from build123d import *

# Parameters (mm, degrees)
SKETCH1_R               = 2.2098
BOSS_EXTRUDE1_DEPTH     = 12.573
CUT_EXTRUDE1_DEPTH      = 3.429
CUT_EXTRUDE1_DEPTH_BACK = 59.054456093
CUT_EXTRUDE5_DEPTH      = 59.054456093
CUT_EXTRUDE5_DEPTH_BACK = 59.054456093
CUT_EXTRUDE6_DEPTH      = 59.054456093
CUT_EXTRUDE6_DEPTH_BACK = 59.054456093
CUT_EXTRUDE7_DEPTH      = 68.574150882
CUT_EXTRUDE7_DEPTH_BACK = 42.0878
FILLET4_R               = 5.715
CUT_EXTRUDE8_START      = 59.054456093
SKETCH11_R              = 2.2098
CUT_EXTRUDE8_DEPTH      = 63.829656093
FILLET5_R               = 0.8128
FILLET6_R               = 0.8128


with BuildPart() as part:
    # Sketch1 → Boss-Extrude1 (new body)
    with BuildSketch(Plane(origin=(0, 0, 0), x_dir=(1, 0, 0), z_dir=(0, 1, 0))):
        with BuildLine():
            Line((-31.5087, -42.4942), (31.5087, -42.4942))
            ThreePointArc((31.5087, -42.4942), (35.747380889, -40.738480889), (37.5031, -36.4998))
            Line((37.5031, -36.4998), (37.5031, 36.4998))
            ThreePointArc((37.5031, 36.4998), (35.747380889, 40.738480889), (31.5087, 42.4942))
            Line((31.5087, 42.4942), (-31.5087, 42.4942))
            ThreePointArc((-31.5087, 42.4942), (-35.747380889, 40.738480889), (-37.5031, 36.4998))
            Line((-37.5031, 36.4998), (-37.5031, -36.4998))
            ThreePointArc((-37.5031, -36.4998), (-35.747380889, -40.738480889), (-31.5087, -42.4942))
        make_face()
        with Locations(Location((-31.5087, 36.4998, 0), (0, 0, 270))):
            Circle(SKETCH1_R, mode=Mode.SUBTRACT)
        with Locations(Location((31.5087, 36.4998, 0), (0, 0, 270))):
            Circle(SKETCH1_R, mode=Mode.SUBTRACT)
        with Locations(Location((31.5087, -36.4998, 0), (0, 0, 270))):
            Circle(SKETCH1_R, mode=Mode.SUBTRACT)
        with Locations(Location((-31.5087, -36.4998, 0), (0, 0, 270))):
            Circle(SKETCH1_R, mode=Mode.SUBTRACT)
    extrude(amount=BOSS_EXTRUDE1_DEPTH)

    # Sketch2 → Cut-Extrude1 (cut, two sides: drawn at the far end of the back side and taken through both)
    with BuildSketch(Plane(origin=(0, 0, 0), x_dir=(1, 0, 0), z_dir=(0, 1, 0)).offset(-CUT_EXTRUDE1_DEPTH_BACK)):
        with BuildLine():
            Line((-6.5024, -42.4942), (3.9624, -42.4942))
            Line((3.9624, -42.4942), (3.9624, 8.7122))
            ThreePointArc((3.9624, 8.7122), (3.843368196, 8.999568196), (3.556, 9.1186))
            Line((3.556, 9.1186), (-6.096, 9.1186))
            ThreePointArc((-6.096, 9.1186), (-6.383368196, 8.999568196), (-6.5024, 8.7122))
            Line((-6.5024, 8.7122), (-6.5024, -42.4942))
        make_face()
    extrude(amount=CUT_EXTRUDE1_DEPTH + CUT_EXTRUDE1_DEPTH_BACK, mode=Mode.SUBTRACT)

    # Sketch8 → Cut-Extrude5 (cut, two sides: drawn at the far end of the back side and taken through both)
    with BuildSketch(Plane.XZ.offset(-CUT_EXTRUDE5_DEPTH_BACK)):
        with BuildLine():
            Line((-6.5024, 42.4942), (3.9624, 42.4942))
            Line((3.9624, 42.4942), (3.9624, 34.9504))
            ThreePointArc((3.9624, 34.9504), (3.843368196, 34.663031804), (3.556, 34.544))
            Line((3.556, 34.544), (-6.096, 34.544))
            ThreePointArc((-6.096, 34.544), (-6.383368196, 34.663031804), (-6.5024, 34.9504))
            Line((-6.5024, 34.9504), (-6.5024, 42.4942))
        make_face()
    extrude(amount=CUT_EXTRUDE5_DEPTH + CUT_EXTRUDE5_DEPTH_BACK, mode=Mode.SUBTRACT)

    # Sketch9 → Cut-Extrude6 (cut, two sides: drawn at the far end of the back side and taken through both)
    with BuildSketch(Plane.XZ.offset(-CUT_EXTRUDE6_DEPTH_BACK)):
        with BuildLine():
            Line((-8.0772, -12.2936), (5.5372, -12.2936))
            ThreePointArc((5.5372, -12.2936), (6.668712271, -11.824912271), (7.1374, -10.6934))
            Line((7.1374, -10.6934), (7.1374, 0.967265238))
            ThreePointArc((7.1374, 0.967265238), (8.243209305, 6.150386126), (11.368068053, 10.430901768))
            Line((11.368068053, 10.430901768), (35.506224679, 32.032963558))
            ThreePointArc((35.506224679, 32.032963558), (36.981158008, 34.053366941), (37.5031, 36.4998))
            Line((37.5031, 36.4998), (37.5031, -42.4942))
            Line((37.5031, -42.4942), (-37.5031, -42.4942))
            Line((-37.5031, -42.4942), (-37.5031, 36.4998))
            ThreePointArc((-37.5031, 36.4998), (-37.04680347, 34.205842433), (-35.747380889, 32.261119111))
            Line((-35.747380889, 32.261119111), (-12.842144818, 9.35588304))
            ThreePointArc((-12.842144818, 9.35588304), (-10.494897301, 5.450135926), (-9.6774, 0.967265238))
            Line((-9.6774, 0.967265238), (-9.6774, -10.6934))
            ThreePointArc((-9.6774, -10.6934), (-9.208712271, -11.824912271), (-8.0772, -12.2936))
        make_face()
    extrude(amount=CUT_EXTRUDE6_DEPTH + CUT_EXTRUDE6_DEPTH_BACK, mode=Mode.SUBTRACT)

    # Sketch10 → Cut-Extrude7 (cut, two sides: drawn at the far end of the back side and taken through both)
    with BuildSketch(Plane(origin=(0, 0, -12.2936), x_dir=(-1, 0, 0), z_dir=(0, 0, -1)).offset(-CUT_EXTRUDE7_DEPTH_BACK)):
        with BuildLine():
            Line((-25.4, 12.573), (25.4, 12.573))
            Line((25.4, 12.573), (25.4, 12.065))
            ThreePointArc((25.4, 12.065), (23.726115254, 8.023884746), (19.685, 6.35))
            Line((19.685, 6.35), (-19.685, 6.35))
            ThreePointArc((-19.685, 6.35), (-23.726115254, 8.023884746), (-25.4, 12.065))
            Line((-25.4, 12.065), (-25.4, 12.573))
        make_face()
    extrude(amount=CUT_EXTRUDE7_DEPTH + CUT_EXTRUDE7_DEPTH_BACK, mode=Mode.SUBTRACT)

    # Fillet4
    fillet4_edges = [part.edges().sort_by_distance(p)[0] for p in [
        (-25.4, 12.319, 29.7942),
        (-23.726115254, 8.023884746, 29.7942),
        (25.4, 12.319, 29.7942),
        (23.726115254, 8.023884746, 29.7942),
        (0, 6.35, 29.7942),
    ]]
    fillet(fillet4_edges, radius=FILLET4_R)

    # Sketch11 → Cut-Extrude8 (cut)
    # profile 1 of 3: a face of its own
    with BuildSketch(Plane.XZ.offset(CUT_EXTRUDE8_START)):
        with BuildLine():
            Line((-37.5031, 22.028038222), (-31.5087, 28.022438222))
            Line((-31.5087, 28.022438222), (-35.747380889, 32.261119111))
            ThreePointArc((-35.747380889, 32.261119111), (-37.04680347, 34.205842433), (-37.5031, 36.4998))
            Line((-37.5031, 36.4998), (-37.5031, 22.028038222))
        make_face()
    # profile 2 of 3: a face of its own
    with BuildSketch(Plane.XZ.offset(CUT_EXTRUDE8_START)):
        with BuildLine():
            ThreePointArc((-27.270019111, 32.261119111), (-25.97059653, 34.205842433), (-25.5143, 36.4998))
            Line((-25.5143, 36.4998), (-25.5143, 42.4942))
            Line((-25.5143, 42.4942), (-31.5087, 42.4942))
            ThreePointArc((-31.5087, 42.4942), (-35.747380889, 40.738480889), (-37.5031, 36.4998))
            ThreePointArc((-37.5031, 36.4998), (-37.04680347, 34.205842433), (-35.747380889, 32.261119111))
            Line((-35.747380889, 32.261119111), (-31.5087, 28.022438222))
            Line((-31.5087, 28.022438222), (-27.270019111, 32.261119111))
        make_face()
        with Locations(Location((-31.5087, 36.4998, 0), (0, 0, 270))):
            Circle(SKETCH11_R, mode=Mode.SUBTRACT)
    # profile 3 of 3: a face of its own
    with BuildSketch(Plane.XZ.offset(CUT_EXTRUDE8_START)):
        with BuildLine():
            ThreePointArc((-37.5031, 36.4998), (-35.747380889, 40.738480889), (-31.5087, 42.4942))
            Line((-31.5087, 42.4942), (-37.5031, 42.4942))
            Line((-37.5031, 42.4942), (-37.5031, 36.4998))
        make_face()
    cut_extrude8 = extrude(amount=-CUT_EXTRUDE8_DEPTH, mode=Mode.SUBTRACT)

    # Mirror1: Cut-Extrude8 across plane
    add(cut_extrude8.mirror(Plane(origin=(0, 0, 0), x_dir=(0, 0, 1), z_dir=(1, 0, 0))), mode=Mode.SUBTRACT)

    # Fillet5
    fillet5_edges = [part.edges().sort_by_distance(p)[0] for p in [
        (-29.389359555, 4.7752, 30.141778666),
        (-25.97059653, 4.7752, 34.205842433),
        (-25.5143, 4.7752, 39.497),
        (29.275106564, 4.7752, 30.256031658),
        (25.97059653, 4.7752, 34.205842433),
        (25.5143, 4.7752, 39.497),
    ]]
    fillet(fillet5_edges, radius=FILLET5_R)

    # Fillet6
    fillet6_edges = [part.edges().sort_by_distance(p)[0] for p in [
        (-6.5024, 6.2865, 42.4942),
        (3.9624, 6.2865, 42.4942),
    ]]
    fillet(fillet6_edges, radius=FILLET6_R)


solid = part.part
Can you work these out from the model? Positions are in its coordinate system, mm. A direction names the side the tool comes from. Round coordinates to 2 decimals unless told otherwise and drop trailing zeros. Order: outer loops, then holes, each group sorted by start corner. A loop starts at its lowest first (then second) coordinate and runs counter-clockwise, first axis right, second up. Notation, with made-up numbers: (73, 63) - (94, 63) arc R20 ccw to (94, 94) - close; hole circle Ø6 at (29.25, -18). An arc over 180 degrees is marked (long way). Answer in a Markdown table with one row per item.
(1) Please list where these lines run through material, in increasing order: L1, parallel to Y at x = -9, z = 16.5; L2, parallel to Z at x = 31.5, y = 5; L3, parallel to X at y = 4.75, z = -0.5. Write a range as from..to.
From the geometry:
| item | result |
|---|---|
| L1 | y = 0..6.35 |
| L2 | z = 28.45..34.29, 38.71..42.49 |
| L3 | x = -9.68..7.14 |
(2) For P1, Ø1, axis at x = -1.5, y = 1, coming from the +Z side; P2, Ø4, axis at y = 10, z = 31.5, coming from the -X side; P3, Ø4.5, axis at x = -3.5, y = 8.5, coming from the +Z side; P4, Ø4, axis at x = 31.51, z = 36.5, coming from the -Y side (1 decimal), each with a flat end and sliding along its axis, tell me the tip position at first contact or that it passes through.
From the geometry:
| item | result |
|---|---|
| P1 | stops at z = -9.12 |
| P2 | stops at x = -36.7 |
| P3 | stops at z = 34.54 |
| P4 | passes through |
(3) Suppose I cut it at B-B, the plane y = 9.25. Please give me the cut outline in (x, z) (3 decimals), plus the area to 3 significant figures.
From the geometry:
| item | result |
|---|---|
| outline | (-35.747, 32.261) - (-24.659, 21.172) - (-24.659, 24.079) arc R4.974 cw to (-19.685, 29.053) - (19.685, 29.053) arc R4.974 cw to (24.659, 24.079) - (24.659, 22.325) - (35.506, 32.033) arc R5.994 ccw to (31.509, 42.494) - (4.775, 42.494) arc R0.813 ccw to (3.962, 41.681) - (3.962, 34.95) arc R0.406 cw to (3.556, 34.544) - (-6.096, 34.544) arc R0.406 cw to (-6.502, 34.95) - (-6.502, 41.681) arc R0.813 ccw to (-7.315, 42.494) - (-31.509, 42.494) arc R5.994 ccw to start; hole circle Ø4.42 at (-31.509, 36.5); hole circle Ø4.42 at (31.509, 36.5) |
| area | 919 mm2 |
(4) Which directions (+Z, -Z, +X, -X, +Y, -Y) give clear straight access to the entire face, cutting with the end or side of a thin tool? Please do faces 5 (the face through (23.77, 12.323, 28.076)), 6 (the face through (3.962, 3, 22)), 7 (the face through (-25.98, 1.95, 34.18)), 8 (the face through (-9.677, 3, -5)).
From the geometry:
| item | result |
|---|---|
| face 5 | -Z, +Y |
| face 6 | +Z, -Y |
| face 7 | +Z, -X, -Y |
| face 8 | -Z, -X, +Y, -Y |
(5) Suppose I cut it at D-D, the plane y = 1. Please give me the cut outline in (x, z).
From the geometry:
| item | result |
|---|---|
| outline | (-31.51, 28.02) - (-12.84, 9.36) arc R12.7 cw to (-9.68, 0.97) - (-9.68, -10.69) arc R1.6 ccw to (-8.08, -12.29) - (5.54, -12.29) arc R1.6 ccw to (7.14, -10.69) - (7.14, 0.97) arc R12.7 cw to (11.37, 10.43) - (31.28, 28.25) - (27.27, 32.26) arc R5.99 cw to (25.51, 36.5) - (25.51, 42.49) - (4.78, 42.49) arc R0.81 ccw to (3.96, 41.68) - (3.96, -8.71) arc R0.41 cw to (3.56, -9.12) - (-6.1, -9.12) arc R0.41 cw to (-6.5, -8.71) - (-6.5, 41.68) arc R0.81 ccw to (-7.32, 42.49) - (-25.51, 42.49) - (-25.51, 36.5) arc R5.99 cw to (-27.27, 32.26) - close |
(6) Suppose I cut it at C-C, the plane x = -0.5. Please give me the cut outline in (y, z) (3 decimals).
From the geometry:
| item | result |
|---|---|
| outline | (0, -12.294) - (6.35, -12.294) - (6.35, 24.079) arc R5.715 cw to (12.065, 29.794) - (12.573, 29.794) - (12.573, 34.544) - (3.429, 34.544) - (3.429, -9.119) - (0, -9.119) - close |
(7) If we mould it in two halves opening along X, with no side actions, what happens to faces 1 (the face through (33.7, 8.6, 36.2)), 2 (the face through (25.95, 4.98, 23.48)), 3 (the face through (-9, 3, -12)), 4 (the face through (-1, 3.429, 13))? For each: released by +X, released by -X, zero draft, split by the parting line, or undercut.
From the geometry:
| item | result |
|---|---|
| face 1 | undercut |
| face 2 | released by +X |
| face 3 | released by -X |
| face 4 | undercut |
(8) Suppose I cut it at A-A, the plane z = -1. Please give me the cut outline in (x, y), plus the area to 3 significant figures.
From the geometry:
| item | result |
|---|---|
| outline | (-9.68, 0) - (-6.5, 0) - (-6.5, 3.43) - (3.96, 3.43) - (3.96, 0) - (7.14, 0) - (7.14, 6.35) - (-9.68, 6.35) - close |
| area | 70.9 mm2 |
